from build123d import *

# Parameters (mm, degrees)
INTEGRATED_START                              = 53
INTEGRATED_HORIZONTAL_STOP_PAD_PROFILE_W      = 16
INTEGRATED_HORIZONTAL_STOP_PAD_PROFILE_H      = 5
INTEGRATED_HORIZONTAL_STOP_PAD_DEPTH          = 4
INTEGRAL_START                                = 53
INTEGRAL_UPRIGHT_PROFILE_W                    = 14
INTEGRAL_UPRIGHT_PROFILE_H                    = 9.7
INTEGRAL_UPRIGHT_DEPTH                        = 4
HORIZONTAL_START                              = 46.65
HORIZONTAL_LIMIT_PIN_ARM_PROFILE_W            = 14
HORIZONTAL_LIMIT_PIN_ARM_PROFILE_H            = 5
HORIZONTAL_LIMIT_PIN_ARM_DEPTH                = 6.55
BUILT_START                                   = 43.35
BUILT_IN_STOP_PIN_DIAMETER_4_MM_PROFILE_R     = 2
BUILT_IN_STOP_PIN_DIAMETER_4_MM_DEPTH         = 3.5
STOP_START                                    = 52.9
STOP_CLEARANCE_TWO_M3_HOLES_10_MM_PI_2_R      = 1.6
STOP_CLEARANCE_TWO_M3_HOLES_10_MM_PITCH_DEPTH = 4.2


with BuildPart() as part:
    # Integrated horizontal stop pad profile → Integrated horizontal stop pad (new body)
    with BuildSketch(Plane.XY.offset(INTEGRATED_START)):
        with Locations((0, 26.5)):
            Rectangle(INTEGRATED_HORIZONTAL_STOP_PAD_PROFILE_W, INTEGRATED_HORIZONTAL_STOP_PAD_PROFILE_H)
    extrude(amount=INTEGRATED_HORIZONTAL_STOP_PAD_DEPTH)

    # Integral upright profile → Integral upright (add)
    with BuildSketch(Plane.XY.offset(INTEGRAL_START)):
        with Locations((0, 19.35)):
            Rectangle(INTEGRAL_UPRIGHT_PROFILE_W, INTEGRAL_UPRIGHT_PROFILE_H)
    extrude(amount=INTEGRAL_UPRIGHT_DEPTH)

    # Horizontal limit pin arm profile → Horizontal limit pin arm (add)
    with BuildSketch(Plane.XY.offset(HORIZONTAL_START)):
        with Locations((0, 17)):
            Rectangle(HORIZONTAL_LIMIT_PIN_ARM_PROFILE_W, HORIZONTAL_LIMIT_PIN_ARM_PROFILE_H)
    extrude(amount=HORIZONTAL_LIMIT_PIN_ARM_DEPTH)

    # Built in stop pin diameter 4 mm profile → Built in stop pin diameter 4 mm (add)
    with BuildSketch(Plane.XY.offset(BUILT_START)):
        with Locations(Location((0, 17.5, 0), (0, 0, 90))):
            Circle(BUILT_IN_STOP_PIN_DIAMETER_4_MM_PROFILE_R)
    extrude(amount=BUILT_IN_STOP_PIN_DIAMETER_4_MM_DEPTH)

    # Stop clearance two M3 holes 10 mm pi 2 → Stop clearance two M3 holes 10 mm pitch (cut)
    with BuildSketch(Plane.XY.offset(STOP_START)):
        with Locations((-5, 27)):
            Circle(STOP_CLEARANCE_TWO_M3_HOLES_10_MM_PI_2_R)
        with Locations((5, 27)):
            Circle(STOP_CLEARANCE_TWO_M3_HOLES_10_MM_PI_2_R)
    extrude(amount=STOP_CLEARANCE_TWO_M3_HOLES_10_MM_PITCH_DEPTH, mode=Mode.SUBTRACT)


solid = part.part
Here's how the part is built. I have some questions about the finished solid (model axes, mm). A direction names the side the tool comes from. Round coordinates to 2 decimals unless told otherwise and drop trailing zeros. Loops run counter-clockwise (first coordinate to the right, second up) from the corner with the lowest first, then second, coordinate; pieces in that order, holes last. Notation, with made-up numbers: M -5.75,-4.75 L 40.25,-4.75 A5 ccw 40.25,4.25 Z; hole C -12,45 d4. An arc over 180 degrees is marked long. Write each question's results on one line, items separated by ' | '. Start each with the question number.
(1) If I drill on probe 1 along X at (y, z) = (27, 54.9); probe 2 along Y at (x, z) = (-5, 55.45); probe 3 along Y at (x, z) = (2.75, 47.5), over which ranges is the centre line in solid material (lowest first)? Write a range as from..to.
(2) I want a section at D-D (x = -3). Please give me the cut outline in (y, z).
(3) I want a section at A-A (y = 27). Please give me the cut outline in (x, z), then the cut area to 3 significant figures.
(4) I want a section at B-B (x = -5). Please give me the cut outline in (y, z), then the cut area to 4 significant figures.
(5) Will these pins go through, and if not, where does the flat tip stop? P1, Ø5, axis at y = 20, z = 52.5, coming from the +X side; P2, Ø5, axis at y = 22.5, z = 50, coming from the -X side; P3, Ø4, axis at y = 21, z = 53, coming from the -X side; P4, Ø2, axis at y = 16.5, z = 45, coming from the +X side.
(6) On a 3-axis mill with a long thin cutter (end or side, diameter ignored), from which of +Z, -Z, +X, -X, +Y, -Y can I reach the whole of each face in a straight line? I mean faces 4 (the flat face through (0, 24, 53)), 5 (the flat face through (-7, 18, 53)), 6 (the cylindrical face through (1.2, 15.9, 45)), 7 (the flat face through (7, 18, 53)), 8 (the flat face through (0, 22, 57)). Say none if no direction works.
(7) Thinking about a two-plate mould opening in Y: for faces 1 (the flat face through (0, 15, 46.65)), 2 (the flat face through (0, 19.5, 50)), 3 (the cylindrical face through (-5.208, 28.586, 54.972)), which applies, pulls with the +Y half, pulls with the -Y half, needs draft (parallel to the pull), parting line crosses it, or undercut?
(8) I want a section at C-C (y = 17.5). Please give me the cut outline in (x, z).
Solved:
1) probe 1: x = -8..-6.6, -3.4..3.4, 6.6..8 | probe 2: y = 14.5..25.4, 28.6..29 | probe 3: y = 14.5..19.5
2) outline: M 14.5,46.65 L 19.5,46.65 L 19.5,53 L 29,53 L 29,57 L 14.5,57 Z
3) outline: M -8,53 L -6.6,53 L -6.6,57 L -8,57 Z; M -3.4,53 L 3.4,53 L 3.4,57 L -3.4,57 Z; M 6.6,53 L 8,53 L 8,57 L 6.6,57 Z | area: 38.4 mm²
4) outline: M 14.5,46.65 L 19.5,46.65 L 19.5,53 L 25.4,53 L 25.4,57 L 14.5,57 Z; M 28.6,53 L 29,53 L 29,57 L 28.6,57 Z | area: 76.95 mm²
5) P1: stops at x = 7 | P2: passes through | P3: stops at x = -7 | P4: stops at x = 2
6) face 4: -Z, +X, -X, +Y | face 5: +Z, -Z, -X, -Y | face 6: -Z | face 7: +Z, -Z, +X, -Y | face 8: +Z, +X, -X, +Y, -Y
7) face 1: needs draft | face 2: pulls with the +Y half | face 3: undercut
8) outline: M -7,46.65 L -2,46.65 L -2,43.35 L 2,43.35 L 2,46.65 L 7,46.65 L 7,57 L -7,57 Z
